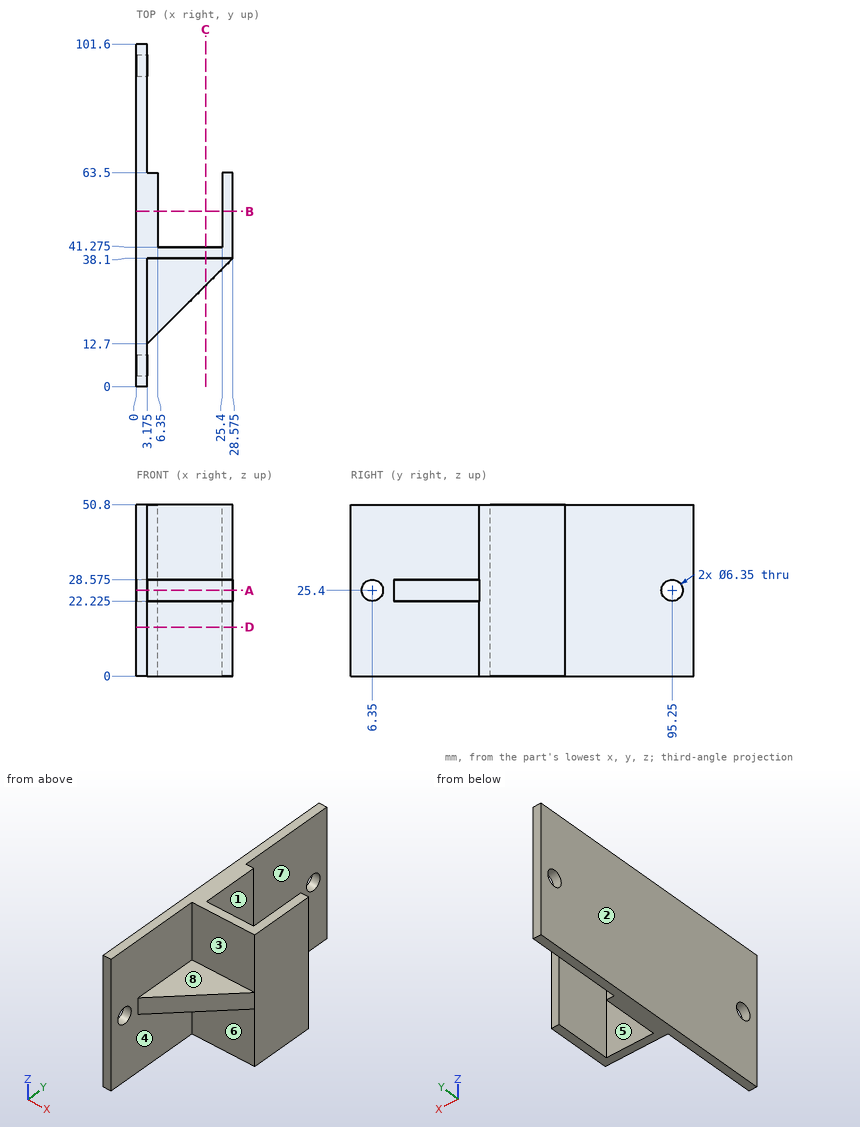
Source: three-view drawing plus pictorial views. Frame: mm from the lowest corner of the part. A direction names the side the tool comes from. Coordinates: 2 decimals unless noted, no trailing zeros. Loops run counter-clockwise (first coordinate to the right, second up) from the corner with the lowest first, then second, coordinate; pieces in that order, holes last. Notation, with made-up numbers: (1.5, -9) - (9.5, -9) arc R18 cw to (9.5, -3) - close; hole circle Ø6 at (78.25, 87.5). An arc over 180 degrees is marked (long way). One line per question, with ' | ' between items.
1) Set-up query: the marked faces 5, 6, 7 and 8. Return all of +Z, -Z, +X, -X, +Y, -Y with unobstructed straight access to the full face (end or side cutting, diameter ignored); none if empty.
Report:
face 5: +Z, -Z, +Y | face 6: -Z, +X, -Y | face 7: +Z, -Z, +X, +Y | face 8: +Z, +X, -Y
2) Section B-B, the plane y = 52. Return loops of the section in (x, z) (3 decimals), then the cut area to 3 significant figures.
Report:
outline: (0, 0) - (6.35, 0) - (6.35, 50.8) - (0, 50.8) - close; (25.4, 0) - (28.575, 0) - (28.575, 50.8) - (25.4, 50.8) - close | area: 484 mm²
3) Section A-A, the plane z = 25.4. Return loops of the section in (x, y) (3 decimals).
Report:
outline: (0, 0) - (3.175, 0) - (3.175, 3.175) - (0, 3.175) - close; (0, 9.525) - (3.175, 9.525) - (3.175, 12.7) - (28.575, 38.1) - (28.575, 63.5) - (25.4, 63.5) - (25.4, 41.275) - (6.35, 41.275) - (6.35, 63.5) - (3.175, 63.5) - (3.175, 92.075) - (0, 92.075) - close; (0, 98.425) - (3.175, 98.425) - (3.175, 101.6) - (0, 101.6) - close
4) Line query: line 1 along Y through (x, z) = (1.7, 25.4) (3 decimals); line 2 along X through (y, z) = (52.5, 11.5) (3 decimals); line 3 along Z through (x, y) = (2, 95.25) (3 decimals). Output: solid intervals per line, ascending.
Report:
line 1: y = 0 to 3.175, 9.525 to 92.075, 98.425 to 101.6 | line 2: x = 0 to 6.35, 25.4 to 28.575 | line 3: z = 0 to 22.225, 28.575 to 50.8
5) First-contact query: P1, Ø3.5, axis at x = 4.5, z = 14, coming from the +Y side; P2, Ø3, axis at x = 21, z = 20.5, coming from the -Y side; P3, Ø2.5, axis at x = 27.5, z = 13.5, coming from the +Y side; P4, Ø1.5, axis at x = 24.5, z = 30, coming from the +Y side (3 decimals). Flat tips, straight axial feed; report the tip coordinate or a pass-through.
Report:
P1: stops at y = 101.6 | P2: stops at y = 38.1 | P3: stops at y = 63.5 | P4: stops at y = 41.275
6) Section C-C, the plane x = 20.5. Return loops of the section in (y, z) (3 decimals), then the cut area to 3 significant figures.
Report:
outline: (30.025, 22.225) - (38.1, 22.225) - (38.1, 0) - (41.275, 0) - (41.275, 50.8) - (38.1, 50.8) - (38.1, 28.575) - (30.025, 28.575) - close | area: 213 mm²
7) Section D-D, the plane z = 14.5. Return loops of the section in (x, y) (3 decimals), then the cut area to 3 significant figures.
Report:
outline: (0, 0) - (3.175, 0) - (3.175, 38.1) - (28.575, 38.1) - (28.575, 63.5) - (25.4, 63.5) - (25.4, 41.275) - (6.35, 41.275) - (6.35, 63.5) - (3.175, 63.5) - (3.175, 101.6) - (0, 101.6) - close | area: 544 mm²
8) Pull-direction query (X, two-part tool) for the marked faces 1, 2, 3 and 4; classes: released by +X, released by -X, zero draft, split by the parting line, or undercut.
Report:
face 1: undercut | face 2: released by -X | face 3: zero draft | face 4: released by +X
